Can you work these out from the model? Positions are in its coordinate system, mm. A direction names the side the tool comes from. Coordinates: 2 decimals unless noted, no trailing zeros. Order: outer loops, then holes, each group sorted by start corner. A loop starts at its lowest first (then second) coordinate and runs counter-clockwise, first axis right, second up.
```python
from build123d import *

# Parameters (mm, degrees)
F1_DEPTH = 72
F2_DEPTH = 6
F4_DEPTH = 70


with BuildPart() as f1:
    # F0 (on Top) → F1 (new body)
    with BuildSketch(Plane.XY):
        with BuildLine():
            Line((98.917353, 93.475991), (-119.482647, 93.475991))
            ThreePointArc((-119.482647, 93.475991), (-134.331889, 87.325233), (-140.482647, 72.475991))
            Line((-140.482647, 72.475991), (-140.482647, -52.724009))
            ThreePointArc((-140.482647, -52.724009), (-134.331889, -67.573252), (-119.482647, -73.724009))
            Line((-119.482647, -73.724009), (98.917353, -73.724009))
            ThreePointArc((98.917353, -73.724009), (113.766596, -67.573252), (119.917353, -52.724009))
            Line((119.917353, -52.724009), (119.917353, 72.475991))
            ThreePointArc((119.917353, 72.475991), (113.766596, 87.325233), (98.917353, 93.475991))
        make_face()
    extrude(amount=-F1_DEPTH)

    # F0 (on Top) → F2 (join)
    with BuildSketch(Plane.XY):
        with BuildLine():
            Line((99.717353, 96.275991), (-120.282647, 96.275991))
            ThreePointArc((-120.282647, 96.275991), (-136.546103, 89.539446), (-143.282647, 73.275991))
            Line((-143.282647, 73.275991), (-143.282647, -56.724009))
            ThreePointArc((-143.282647, -56.724009), (-136.546103, -72.987465), (-120.282647, -79.724009))
            Line((-120.282647, -79.724009), (99.717353, -79.724009))
            ThreePointArc((99.717353, -79.724009), (115.980809, -72.987465), (122.717353, -56.724009))
            Line((122.717353, -56.724009), (122.717353, 73.275991))
            ThreePointArc((122.717353, 73.275991), (115.980809, 89.539446), (99.717353, 96.275991))
        make_face()
        with BuildLine():
            ThreePointArc((-140.482647, 72.475991), (-134.331889, 87.325233), (-119.482647, 93.475991))
            Line((-119.482647, 93.475991), (98.917353, 93.475991))
            ThreePointArc((98.917353, 93.475991), (113.766596, 87.325233), (119.917353, 72.475991))
            Line((119.917353, 72.475991), (119.917353, -52.724009))
            ThreePointArc((119.917353, -52.724009), (113.766596, -67.573252), (98.917353, -73.724009))
            Line((98.917353, -73.724009), (-119.482647, -73.724009))
            ThreePointArc((-119.482647, -73.724009), (-134.331889, -67.573252), (-140.482647, -52.724009))
            Line((-140.482647, -52.724009), (-140.482647, 72.475991))
        make_face(mode=Mode.SUBTRACT)
    extrude(amount=-F2_DEPTH)

    # F3 (on face) → F4 (cut)
    with BuildSketch(Plane.XY):
        with BuildLine():
            Line((98.917353, 92.975991), (-119.482647, 92.975991))
            ThreePointArc((-119.482647, 92.975991), (-133.978336, 86.97168), (-139.982647, 72.475991))
            Line((-139.982647, 72.475991), (-139.982647, -52.724009))
            ThreePointArc((-139.982647, -52.724009), (-133.978336, -67.219699), (-119.482647, -73.224009))
            Line((-119.482647, -73.224009), (98.917353, -73.224009))
            ThreePointArc((98.917353, -73.224009), (113.413042, -67.219699), (119.417353, -52.724009))
            Line((119.417353, -52.724009), (119.417353, 72.475991))
            ThreePointArc((119.417353, 72.475991), (113.413042, 86.97168), (98.917353, 92.975991))
        make_face()
    extrude(amount=-F4_DEPTH, mode=Mode.SUBTRACT)


solid = f1.part
```
1. I'm going to push flat-ended pins straight in: pin 1 (8 mm diameter, centred on y = -4, z = -49, fed in from -X); pin 2 (3 mm diameter, centred on y = 40.5, z = -32, fed in from +X); pin 3 (1.5 mm diameter, centred on x = 40.5, z = -48.5, fed in from -Y). Where does each tip first touch, or does it pass through?
Completed:
pin 1: stops at x = -140.48
pin 2: stops at x = 119.92
pin 3: stops at y = -73.72
2. Thinking about a two-plate mould opening in X: for faces 6 (the cylindrical face through (-134.494, -67.409, -38.538)), 7 (the cylindrical face through (113.93, 87.16, -38.54)), 8 (the flat face through (119.417, 9, -35)), 9 (the flat face through (-9, 96.276, -3)), which applies, pulls with the +X half, pulls with the -X half, needs draft (parallel to the pull), parting line crosses it, or undercut?
Completed:
face 6: pulls with the -X half
face 7: pulls with the +X half
face 8: undercut
face 9: needs draft
3. Imagine slicing it at C-C on y = 12. Please give me the cut outline in (x, z), then the cut area to 3 significant figures.
Completed:
outline: (-143.28, -6) - (-140.48, -6) - (-140.48, -72) - (119.92, -72) - (119.92, -6) - (122.72, -6) - (122.72, 0) - (119.42, 0) - (119.42, -70) - (-139.98, -70) - (-139.98, 0) - (-143.28, 0) - close
area: 624 mm2
4. Imagine slicing it at A-A on z = -34. Please give me the cut outline in (x, y), then the cut area to 3 significant figures.
Completed:
outline: (-140.48, -52.72) arc R21 ccw to (-119.48, -73.72) - (98.92, -73.72) arc R21 ccw to (119.92, -52.72) - (119.92, 72.48) arc R21 ccw to (98.92, 93.48) - (-119.48, 93.48) arc R21 ccw to (-140.48, 72.48) - close; hole (-139.98, -52.72) arc R20.5 ccw to (-119.48, -73.22) - (98.92, -73.22) arc R20.5 ccw to (119.42, -52.72) - (119.42, 72.48) arc R20.5 ccw to (98.92, 92.98) - (-119.48, 92.98) arc R20.5 ccw to (-139.98, 72.48) - close
area: 409 mm2
5. Please list where these lines run through material, in increasing order: probe 1 along X at (y, z) = (51.5, -19); probe 2 along Y at (x, z) = (-111.5, -21.5); probe 3 along Y at (x, z) = (-99, -5.5).
Completed:
probe 1: x = -140.48 to -139.98, 119.42 to 119.92
probe 2: y = -73.72 to -73.22, 92.98 to 93.48
probe 3: y = -79.72 to -73.22, 92.98 to 96.28
6. Imagine slicing it at B-B on x = -61.5. Please give me the cut outline in (y, z), then the cut area to 3 significant figures.
Completed:
outline: (-79.72, -6) - (-73.72, -6) - (-73.72, -72) - (93.48, -72) - (93.48, -6) - (96.28, -6) - (96.28, 0) - (92.98, 0) - (92.98, -70) - (-73.22, -70) - (-73.22, 0) - (-79.72, 0) - close
area: 457 mm2
7. On a 3-axis mill with a long thin cutter (end or side, diameter ignored), from which of +Z, -Z, +X, -X, +Y, -Y can I reach the whole of each face in a straight line? I mean faces 1 (the flat face through (-12, -73.724, -39)), 2 (the flat face through (119.917, 9, -39)), 3 (the cylindrical face through (113.6, -67.74, -38.54)), 4 (the cylindrical face through (-133.82, 87.13, -34.51)), 5 (the cylindrical face through (-134.168, 87.488, -38.538)). Say none if no direction works.
Completed:
face 1: -Z, +X, -X, -Y
face 2: -Z, +X, +Y, -Y
face 3: -Z, +X, -Y
face 4: +Z
face 5: -Z, -X, +Y
